```python
from build123d import *

# Parameters (mm, degrees)
SKIZZE2_W  = 1.1
SKIZZE2_H  = 0.2
FASE1_SIZE = 1


with BuildPart() as part:
    # Skizze1 → Rotation1 (revolve)
    with BuildSketch(Plane(origin=(0, 0, 0), x_dir=(1, 0, 0), z_dir=(0, 1, 0))):
        Polygon((-63, -5), (-50, -5), (-50, -7), (50, -7), (50, -5), (63, -5), (63, 0), (-63, 0), align=None)
    revolve(axis=Axis((-125.234019669, 0, 0), (1, 0, 0)))

    # Skizze2 → Schnitt-Rotation1 (revolve, cut)
    with BuildSketch(Plane(origin=(0, 0, 0), x_dir=(1, 0, 0), z_dir=(0, 1, 0))):
        with Locations((58.55, -4.9)):
            Rectangle(SKIZZE2_W, SKIZZE2_H)
        with Locations((-58.55, -4.9)):
            Rectangle(SKIZZE2_W, SKIZZE2_H)
    revolve(axis=Axis((0, 0, 0), (1, 0, 0)), mode=Mode.SUBTRACT)

    # Fase1
    fase1_edges = [part.edges().sort_by_distance(p)[0] for p in [
        (63, 0, -5),
    ]]
    chamfer(fase1_edges, length=FASE1_SIZE)


solid = part.part
```
Model file for the job. Use its own axes, mm. A direction names the side the tool comes from. Give positions to 0.01 mm unless a question says otherwise; leave off trailing zeros. Write each loop counter-clockwise with the first axis right and the second up, starting at its lowest first coordinate (ties: lowest second). Pieces come first, ordered by that corner, then holes. Notation, with made-up numbers: (-37, 27) -> (15, 27) arc R37 ccw to (15, 64) -> close; hole circle Ø5 at (86, 73). An arc over 180 degrees is marked (long way). Use CSV: the item, a comma, the result in double quotes. Start each with the question number.
1) Cut at C-C on x = 35. List the corners of the cut face in (y, z), plus the area to 3 significant figures.
2) Cut at D-D on x = 55.5. List the corners of the cut face in (y, z), plus the area to 3 significant figures.
3) Tool access for faces 1 (the cylindrical face through (54.06, 4.88, -1.08)), 2 (the cylindrical face through (58.56, -4.05, 2.58)), 3 (the flat face through (-50, -5, 2)): list every direction of +Z, -Z, +X, -X, +Y, -Y with a clear straight run to the whole face (end or side of a thin tool).
4) Pin check, flat tips, straight feed: P1, Ø3, axis at x = -29, z = 2.5, coming from the -Y side; P2, Ø6, axis at x = 3, y = 4, coming from the -Z side; P3, Ø8, axis at x = -42, z = 2, coming from the -Y side; P4, Ø1, axis at y = 5, z = 3.5, coming from the -X side. Stop position of each tip, or through.
5) Drill centre lines: L1, parallel to X at y = 5, z = -4.25; L2, parallel to Y at x = 45, z = 0.25; L3, parallel to Y at x = -27, z = 2. Where is each one in solid material? Low to high.
Final values:
1,outline,"circle Ø14 at (0, 0)"
1,area,"154 mm2"
2,outline,"circle Ø10 at (0, 0)"
2,area,"78.5 mm2"
3,face 1,"+X"
3,face 2,"none"
3,face 3,"-X"
4,P1,"stops at y = -6.93"
4,P2,"stops at z = -6.93"
4,P3,"stops at y = -7"
4,P4,"stops at x = -50"
5,L1,"x = -50 to 50"
5,L2,"y = -7 to 7"
5,L3,"y = -6.71 to 6.71"
